Part model, mm, in its own coordinate system. Face numbers are marked on the shaded views. A direction names the side the tool comes from. Coordinates: 2 decimals unless noted, no trailing zeros. Write each loop counter-clockwise with the first axis right and the second up, starting at its lowest first coordinate (ties: lowest second). Pieces come first, ordered by that corner, then holes. Notation, with made-up numbers: (19.5, 67.25) - (33.5, 67.25) arc R17 cw to (33.5, 81.25) - close; hole circle Ø2 at (66, 37). An arc over 180 degrees is marked (long way). Use a Markdown table: item, result.
```python
from build123d import *

# Parameters (mm, degrees)
ESQUISSE2_W             = 60
ESQUISSE2_H             = 60
BOSS_EXTRU_1_DEPTH      = 5
ESQUISSE3_R             = 2
ENL_V_MAT_EXTRU_1_DEPTH = 5
CONG_1_R                = 6
TROU_TARAUD_M51_D       = 4.2
TROU_TARAUD_M51_DEPTH   = 24
TROU_TARAUD_M51_TIP     = 1.2618073


with BuildPart() as part:
    # Esquisse1 → Révolution1 (revolve)
    with BuildSketch(Plane.XY, mode=Mode.PRIVATE) as r_volution1_sk:
        Polygon((0, 0), (28, 0), (28, 65), (16, 65), (16, 67), (6, 67), (6, 95), (0, 95), align=None)
    revolve(r_volution1_sk.sketch.rotate(Axis((0, 0, 0), (0, 1, 0)), 90), axis=Axis((0, 0, 0), (0, 1, 0)))

    # Esquisse2 → Boss.-Extru.1 (add)
    with BuildSketch(Plane.XZ):
        Rectangle(ESQUISSE2_W, ESQUISSE2_H)
    extrude(amount=BOSS_EXTRU_1_DEPTH)

    # Esquisse3 → Enlèv. mat.-Extru.1 (cut)
    with BuildSketch(Plane.XZ.offset(5)):
        with Locations(Location((-23.57, 23.57, 0), (0, 0, 270))):
            Circle(ESQUISSE3_R)
        with Locations(Location((23.57, 23.57, 0), (0, 0, 270))):
            Circle(ESQUISSE3_R)
        with Locations(Location((-23.57, -23.57, 0), (0, 0, 270))):
            Circle(ESQUISSE3_R)
        with Locations(Location((23.57, -23.57, 0), (0, 0, 270))):
            Circle(ESQUISSE3_R)
    extrude(amount=-ENL_V_MAT_EXTRU_1_DEPTH, mode=Mode.SUBTRACT)

    # Congé1
    cong_1_edges = [part.edges().sort_by_distance(p)[0] for p in [
        (-30, -2.5, 30),
        (-30, -2.5, -30),
        (30, -2.5, -30),
        (30, -2.5, 30),
    ]]
    fillet(cong_1_edges, radius=CONG_1_R)

    # Trou taraudé M51
    with Locations(Plane(origin=(0, 65, 0), x_dir=(1, 0, 0), z_dir=(0, 1, 0))):
        with Locations((-16.617009358, 16.617009358), (16.617009358, 16.617009358), (16.617009358, -16.617009358), (-16.617009358, -16.617009358)):
            Hole(TROU_TARAUD_M51_D / 2, depth=TROU_TARAUD_M51_DEPTH)
            with Locations((0, 0, -(TROU_TARAUD_M51_DEPTH + TROU_TARAUD_M51_TIP / 2))):  # 118° drill point
                Cone(0, TROU_TARAUD_M51_D / 2, TROU_TARAUD_M51_TIP, mode=Mode.SUBTRACT)


solid = part.part
```
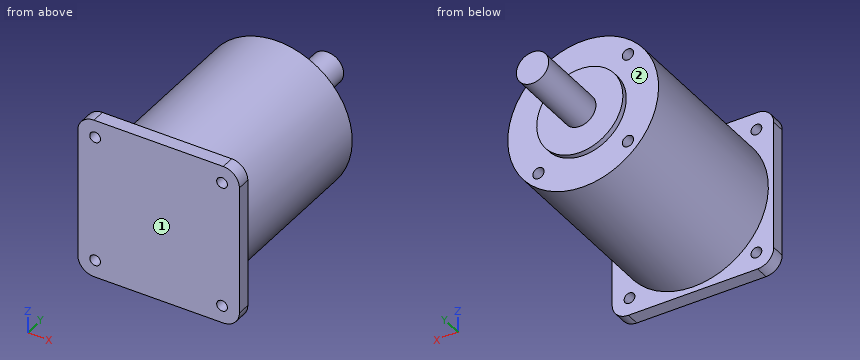
Item 1: Band-saw the part on D-D, the plane y = 29. Give the cut face in (x, z), then the cut area to 3 significant figures.
From the geometry:
| item | result |
|---|---|
| outline | circle Ø56 at (0, 0) |
| area | 2,460 mm^2 |
Item 2: Drop flat-ended pins along their axis: P1, Ø12, axis at x = -8, y = 82, coming from the +Z side; P2, Ø12, axis at y = 63.5, z = 8.5, coming from the -X side; P3, Ø3, axis at x = -23.57, z = -23.57, coming from the +Y side; P4, Ø12, axis at x = -2.5, y = 81, coming from the -Z side. Give the stop position or say it passes through.
From the geometry:
| item | result |
|---|---|
| P1 | z = 5.66 |
| P2 | x = -27.89 |
| P3 | through |
| P4 | z = -6 |
Item 3: Which spindle directions (+Z, -Z, +X, -X, +Y, -Y) get a long thin tool onto all of the face, cutting with end or side? Do the marked faces 1 and 2. Say none if no direction does.
From the geometry:
| item | result |
|---|---|
| face 1 | +Z, -Z, +X, -X, -Y |
| face 2 | +Y |
Item 4: Drill centre lines: probe 1 along X at (y, z) = (-2, -23); probe 2 along X at (y, z) = (63, 16.5). Where is each one in solid material? Low to high.
From the geometry:
| item | result |
|---|---|
| probe 1 | -30 to -25.49, -21.65 to 21.65, 25.49 to 30 |
| probe 2 | -22.62 to -18.71, -14.52 to 14.52, 18.71 to 22.62 |
Item 5: Band-saw the part on B-B, the plane x = 0. Give the cut face in (y, z).
From the geometry:
| item | result |
|---|---|
| outline | (-5, -30) - (0, -30) - (0, -28) - (65, -28) - (65, -16) - (67, -16) - (67, -6) - (95, -6) - (95, 6) - (67, 6) - (67, 16) - (65, 16) - (65, 28) - (0, 28) - (0, 30) - (-5, 30) - close |
Item 6: Band-saw the part on C-C, the plane y = 74. Give the cut face in (x, z), then the cut area to 3 significant figures.
From the geometry:
| item | result |
|---|---|
| outline | circle Ø12 at (0, 0) |
| area | 113 mm^2 |
Item 7: Band-saw the part on A-A, the plane z = 0. Give the cut face in (x, y), then the cut area to 3 significant figures.
From the geometry:
| item | result |
|---|---|
| outline | (-30, -5) - (30, -5) - (30, 0) - (28, 0) - (28, 65) - (16, 65) - (16, 67) - (6, 67) - (6, 95) - (-6, 95) - (-6, 67) - (-16, 67) - (-16, 65) - (-28, 65) - (-28, 0) - (-30, 0) - close |
| area | 4,340 mm^2 |
